```python
from build123d import *

# Parameters (mm, degrees)
SKETCH023_W     = 76
SKETCH023_H     = 30
PAD006_DEPTH    = 4
PAD007_DEPTH    = 76
SKETCH028_R     = 2.75
HOLE004_DEPTH   = 24.001
SKETCH032_R     = 2.75
HOLE005_DEPTH   = 25.001
SKETCH033_W     = 45
SKETCH033_H     = 20
POCKET010_DEPTH = 56.001
POCKET011_DEPTH = 21.001


with BuildPart() as part:
    # Sketch023 → Pad006 (new body)
    with BuildSketch(Plane.XZ):
        with Locations((-170, 200)):
            Rectangle(SKETCH023_W, SKETCH023_H)
    extrude(amount=PAD006_DEPTH)

    # Sketch024 → Pad007 (join)
    with BuildSketch(Plane.YZ.offset(-132)):
        Polygon((0, 215), (0, 210), (17, 210), (17, 228), (13, 228), (13, 215), align=None)
        Polygon((0, 190), (17, 190), (17, 172), (13, 172), (13, 185), (0, 185), align=None)
    extrude(amount=-PAD007_DEPTH)

    # Sketch028 → Hole004 (cut, through all)
    with BuildSketch(Plane(origin=(0, 20, 0), x_dir=(1, 0, 0), z_dir=(0, 1, 0))):
        with Locations((-200, -220)):
            Circle(SKETCH028_R)
        with Locations((-200, -180)):
            Circle(SKETCH028_R)
        with Locations((-140, -180)):
            Circle(SKETCH028_R)
        with Locations((-140, -220)):
            Circle(SKETCH028_R)
    extrude(amount=-HOLE004_DEPTH, mode=Mode.SUBTRACT)

    # Sketch032 → Hole005 (cut, through all)
    with BuildSketch(Plane.XZ.offset(8)):
        with Locations((-190, 200)):
            Circle(SKETCH032_R)
        with Locations((-150, 200)):
            Circle(SKETCH032_R)
    extrude(amount=-HOLE005_DEPTH, mode=Mode.SUBTRACT)

    # Sketch033 (on Face22 of Hole005) → Pocket010 (cut, through all)
    with BuildSketch(Plane(origin=(0, 0, 228), x_dir=(-1, 0, 0), z_dir=(0, 0, 1))):
        with Locations((170, -10)):
            Rectangle(SKETCH033_W, SKETCH033_H)
    extrude(amount=-POCKET010_DEPTH, mode=Mode.SUBTRACT)

    # Sketch034 (on Face7 of Pocket010) → Pocket011 (cut, through all)
    with BuildSketch(Plane.XZ.offset(4)):
        Polygon((-210, 210), (-200, 200), (-210, 190), align=None)
        Polygon((-130, 210), (-140, 200), (-130, 190), align=None)
        Polygon((-192.5, 218), (-147.5, 218), (-170, 206), align=None)
        Polygon((-192.5, 182), (-147.5, 182), (-170, 194), align=None)
    extrude(amount=-POCKET011_DEPTH, mode=Mode.SUBTRACT)


with BuildPart() as part_1:
    # Body004 placement: moved
    add(part.part.moved(Location((0, 119, 0))))


solid = part_1.part
```
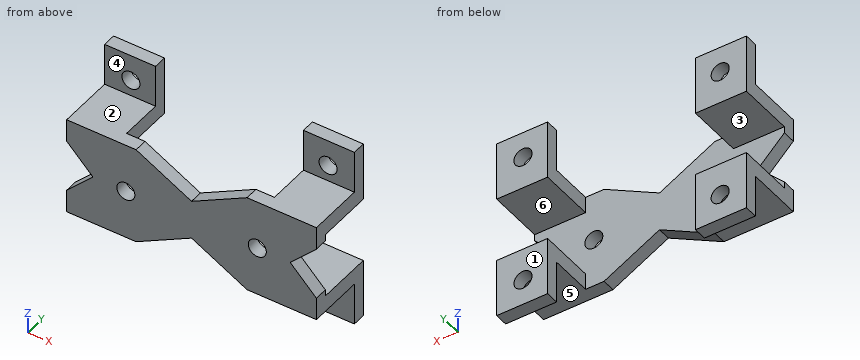
Read the model definition and answer for the solid it produces. Units are mm, in the model's axes. Face numbers are marked on the shaded views. A direction names the side the tool comes from. Give positions to 0.01 mm unless a question says otherwise; leave off trailing zeros. Write each loop counter-clockwise with the first axis right and the second up, starting at its lowest first coordinate (ties: lowest second). Pieces come first, ordered by that corner, then holes. Notation, with made-up numbers: (60, 17.5) -> (65, 17.5) arc R27 ccw to (65, 42.5) -> close; hole circle Ø10 at (16.5, -23). An arc over 180 degrees is marked (long way). Answer in a Markdown table with one row per item.
1) Determine the mould class of the marked faces 1, 2 and 3 for opening direction Z: released by +Z, released by -Z, zero draft, split by the parting line, or undercut.
Results list:
| item | result |
|---|---|
| face 1 | zero draft |
| face 2 | released by +Z |
| face 3 | undercut |
2) A tool of negligible diameter and unlimited length cuts with its end or side. For the marked faces 4, 5 and 6, from which of +Z, -Z, +X, -X, +Y, -Y can it reach the whole face along a straight path? Write none if from no direction.
Results list:
| item | result |
|---|---|
| face 4 | +Z, +X, -X, -Y |
| face 5 | -Z, +X, -X, -Y |
| face 6 | +X, -X, +Y |
3) Section A-A on z = 176 is taken. Give the vertices of the cut face in (x, y), plus the area to 3 significant figures.
Results list:
| item | result |
|---|---|
| outline | (-208, 132) -> (-192.5, 132) -> (-192.5, 136) -> (-208, 136) -> close; (-147.5, 132) -> (-132, 132) -> (-132, 136) -> (-147.5, 136) -> close |
| area | 124 mm^2 |
4) Section D-D on z = 220 is taken. Give the vertices of the cut face in (x, y), plus the area to 3 significant figures.
Results list:
| item | result |
|---|---|
| outline | (-208, 132) -> (-202.75, 132) -> (-202.75, 136) -> (-208, 136) -> close; (-197.25, 132) -> (-192.5, 132) -> (-192.5, 136) -> (-197.25, 136) -> close; (-147.5, 132) -> (-142.75, 132) -> (-142.75, 136) -> (-147.5, 136) -> close; (-137.25, 132) -> (-132, 132) -> (-132, 136) -> (-137.25, 136) -> close |
| area | 80.0 mm^2 |
5) Section C-C on y = 123.5 is taken. Give the vertices of the cut face in (x, z), plus the area to 3 significant figures.
Results list:
| item | result |
|---|---|
| outline | (-208, 185) -> (-192.5, 185) -> (-192.5, 190) -> (-208, 190) -> close; (-208, 210) -> (-192.5, 210) -> (-192.5, 215) -> (-208, 215) -> close; (-147.5, 185) -> (-132, 185) -> (-132, 190) -> (-147.5, 190) -> close; (-147.5, 210) -> (-132, 210) -> (-132, 215) -> (-147.5, 215) -> close |
| area | 310 mm^2 |
6) Section B-B on x = -190 is taken. Give the vertices of the cut face in (y, z), plus the area to 3 significant figures.
Results list:
| item | result |
|---|---|
| outline | (115, 185) -> (119, 185) -> (119, 197.25) -> (115, 197.25) -> close; (115, 202.75) -> (119, 202.75) -> (119, 215) -> (115, 215) -> close |
| area | 98.0 mm^2 |
7) Straight lines are drawn through the part: line 1 (X direction, y = 115.9, z = 200); line 2 (X direction, y = 134.1, z = 180); line 3 (Z direction, x = -200, y = 133.5). For each, find the intervals that lie inside material, in ascending order. Write a range as [from, to].
Results list:
| item | result |
|---|---|
| line 1 | [-200, -192.75], [-187.25, -152.75], [-147.25, -140] |
| line 2 | [-208, -202.75], [-197.25, -192.5], [-147.5, -142.75], [-137.25, -132] |
| line 3 | [172, 177.25], [182.75, 190], [210, 217.25], [222.75, 228] |
8) Each of these flat-tipped pins is pushed along its axis until it touches: pin 1 Ø10.5 at (x, z) = (-200.5, 221.5) entering from -Y; pin 2 Ø8.5 at (x, y) = (-138, 123) entering from +Z; pin 3 Ø1 at (x, z) = (-179.5, 211.5) entering from +Y; pin 4 Ø8 at (x, y) = (-198, 129.5) entering from -Z. Where does it stop, or does it pass through?
Results list:
| item | result |
|---|---|
| pin 1 | y = 132 |
| pin 2 | z = 215 |
| pin 3 | y = 119 |
| pin 4 | z = 172 |
